Part print with two shaded views. Sizes in mm from the minimum x, y, z corner. A direction names the side the tool comes from. Coordinates: 2 decimals unless noted, no trailing zeros. Loops run counter-clockwise (first coordinate to the right, second up) from the corner with the lowest first, then second, coordinate; pieces in that order, holes last.
(1) Slice it at A-A (x = 41). Give the cut face in (y, z), and give its area (3 significant figures).
(2) Wall check: L1, parallel to X at y = 12, z = 4.5; L2, parallel to Y at x = 23, z = 19.5; L3, parallel to Z at x = 53, y = 100. Give the ranges that are in metal, low to high.
(3) Slice it at C-C (z = 50). Give the cut face in (x, y), and give its area (3 significant figures).
(4) Two-plate mould, pull along Y, no slides. Class the marked faces 3, 4 and 5: pulls with the +Y half, pulls with the -Y half, needs draft (parallel to the pull), parting line crosses it, or undercut.
(5) Slice it at B-B (y = 114). Give the cut face in (x, z), and give its area (3 significant figures).
(6) Slice it at D-D (z = 56.5). Give the cut face in (x, y).
(7) Tool access for the marked faces 1 and 2: list every direction of +Z, -Z, +X, -X, +Y, -Y with a clear straight run to the whole face (end or side of a thin tool).
(8) Flat gauge pin, fed straight in: P1, Ø5, axis at x = 34.5, y = 21.5, coming from the +Z side. Where does the tip first touch, or does it go through?
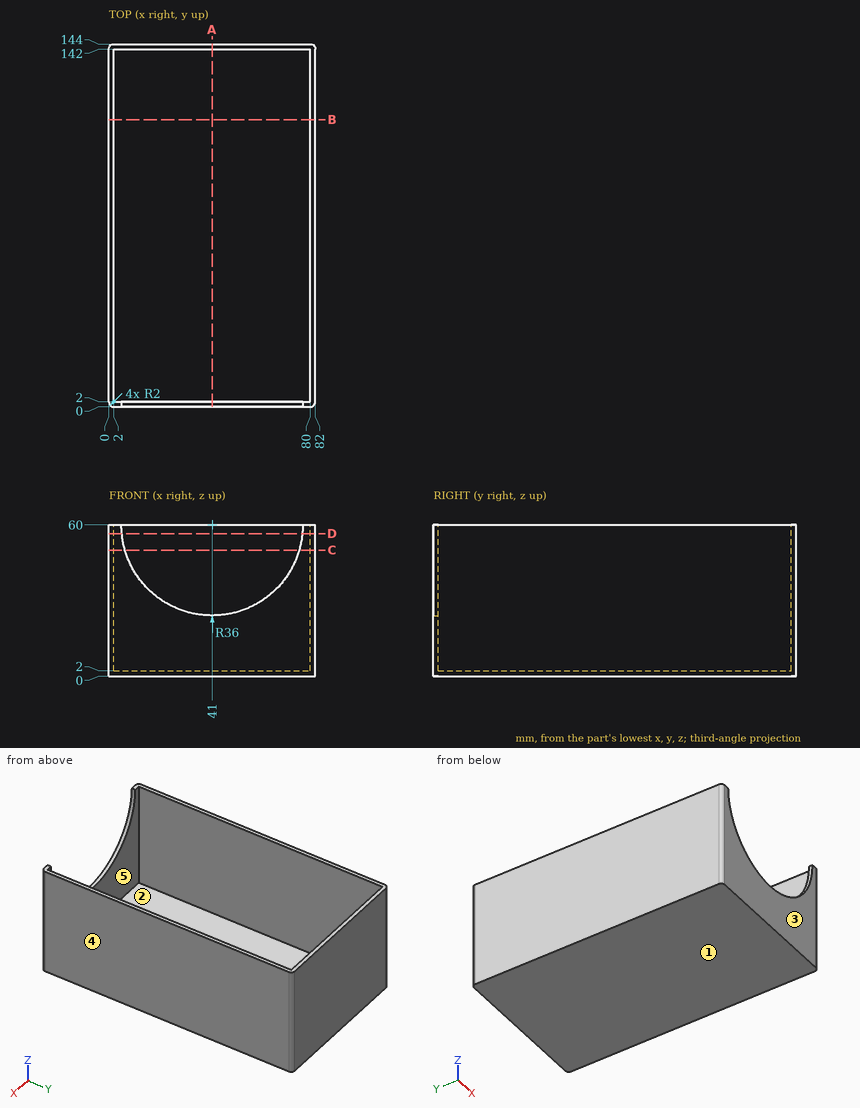
Response values:
1. outline: (0, 0) - (144, 0) - (144, 60) - (142, 60) - (142, 2) - (2, 2) - (2, 24) - (0, 24) - close
1. area: 448 mm2
2. L1: x = 0 to 2, 80 to 82
2. L2: y = 0 to 2, 142 to 144
2. L3: z = 0 to 2
3. outline: (0, 2) arc R2 ccw to (2, 0) - (6.42, 0) - (6.42, 2) - (2, 2) - (2, 142) - (80, 142) - (80, 2) - (75.58, 2) - (75.58, 0) - (80, 0) arc R2 ccw to (82, 2) - (82, 142) arc R2 ccw to (80, 144) - (2, 144) arc R2 ccw to (0, 142) - close
3. area: 746 mm2
4. face 3: pulls with the -Y half
4. face 4: needs draft
4. face 5: undercut
5. outline: (0, 0) - (82, 0) - (82, 60) - (80, 60) - (80, 2) - (2, 2) - (2, 60) - (0, 60) - close
5. area: 396 mm2
6. outline: (0, 2) arc R2 ccw to (2, 0) - (5.17, 0) - (5.17, 2) - (2, 2) - (2, 142) - (80, 142) - (80, 2) - (76.83, 2) - (76.83, 0) - (80, 0) arc R2 ccw to (82, 2) - (82, 142) arc R2 ccw to (80, 144) - (2, 144) arc R2 ccw to (0, 142) - close
7. face 1: -Z, +X, -X, +Y, -Y
7. face 2: +Z
8. P1: stops at z = 2
